Design review of the part built by this model. Coordinates are the model's own, in mm. Face numbers are marked on the shaded views. A direction names the side the tool comes from. Give positions to 0.01 mm unless a question says otherwise; leave off trailing zeros. Order: outer loops, then holes, each group sorted by start corner. A loop starts at its lowest first (then second) coordinate and runs counter-clockwise, first axis right, second up. Notation, with made-up numbers: (2.25, 65) -> (36.25, 65) arc R18 cw to (36.25, 91) -> close; hole circle Ø4 at (66.25, -12). An arc over 180 degrees is marked (long way). Answer in a Markdown table with one row per item. Add a question column.
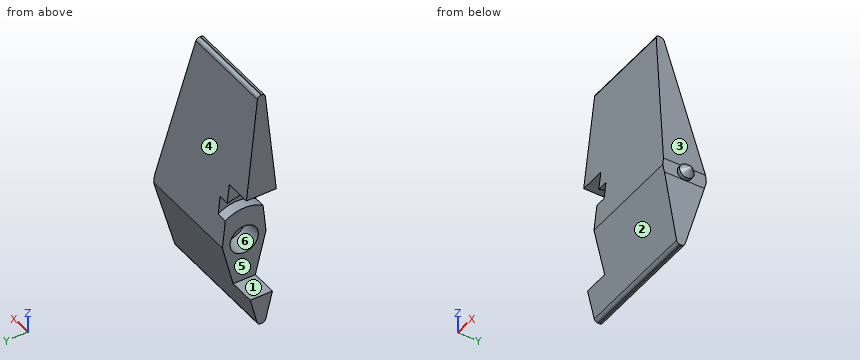
```python
from build123d import *

# Parameters (mm, degrees)
SKETCH_1_3_R                  = 1.95
CUT_EXTRUDE_1_DEPTH           = 6.5
CUT_EXTRUDE_2_DEPTH           = 30.951001802
CUT_EXTRUDE_2_DEPTH_BACK      = 30.951001802
SKETCH_4_W                    = 3.6
SKETCH_4_H                    = 14.9
SKETCH_5_W                    = 1.5
SKETCH_5_H                    = 2.1
CUT_REVOLVE_1_ANGLE           = 40
CUT_REVOLVE_1_OTHER_WAY_ANGLE = 40
SKETCH_3_3_R                  = 1
EXTRUDE_1_DEPTH               = 1.5
CHAMFER_1_SIZE                = 1
CUT_EXTRUDE_3_DEPTH           = 31.875759187
CUT_EXTRUDE_3_DEPTH_BACK      = 31.875759187
FILLET_1_R                    = 0.5


with BuildPart() as part:
    # Эскиз1 → По сечениям1 section 0
    with BuildSketch(Plane(origin=(0, 0, 0), x_dir=(0, 0, -1), z_dir=(1, 0, 0))):
        with BuildLine():
            Line((-23.75, -0.5), (-23.75, 0.5))
            Line((-23.75, 0.5), (0, 3))
            Line((0, 3), (10, 0.5))
            Line((10, 0.5), (10, -0.5))
            Line((10, -0.5), (0, -3))
            Line((0, -3), (-23.75, -0.5))
        make_face()
    # Эскиз3 → По сечениям1 section 1
    with BuildSketch(Plane(origin=(18, 0, 0), x_dir=(0, 0, -1), z_dir=(1, 0, 0))):
        with BuildLine():
            Line((0, 3), (10, 0.5))
            Line((10, 0.5), (10, -0.5))
            Line((10, -0.5), (0, -3))
            Line((0, -3), (-23.75, -0.5))
            Line((-23.75, -0.5), (-23.75, 0.5))
            Line((-23.75, 0.5), (0, 3))
        make_face()
    loft()

    # Эскиз1<3> → Вырез-Вытянуть1 (cut)
    with BuildSketch(Plane(origin=(0, 0, 0), x_dir=(0, 0, -1), z_dir=(1, 0, 0))):
        with Locations(Location((0, 0, 0), (0, 0, 180))):
            Circle(SKETCH_1_3_R)
    extrude(amount=CUT_EXTRUDE_1_DEPTH, mode=Mode.SUBTRACT)

    # Эскиз4 → Вырез-Вытянуть2 (cut, two sides: drawn at the far end of the back side and taken through both)
    with BuildSketch(Plane(origin=(0, 0, 0), x_dir=(1, 0, 0), z_dir=(0, 1, 0)).offset(-CUT_EXTRUDE_2_DEPTH_BACK)):
        with Locations((1.8, -1.55)):
            Rectangle(SKETCH_4_W, SKETCH_4_H)
    extrude(amount=CUT_EXTRUDE_2_DEPTH + CUT_EXTRUDE_2_DEPTH_BACK, mode=Mode.SUBTRACT)

    # Эскиз5 → Вырез-Повернуть1 (revolve, cut)
    with BuildSketch(Plane(origin=(0, 0, 0), x_dir=(1, 0, 0), z_dir=(0, 1, 0))):
        with Locations((4.35, -5.7)):
            Rectangle(SKETCH_5_W, SKETCH_5_H)
    revolve(axis=Axis((6.5, 0, 0), (-1, 0, 0)), revolution_arc=CUT_REVOLVE_1_ANGLE, mode=Mode.SUBTRACT)

    # Эскиз5 → Вырез-Повернуть1 other way (revolve, cut)
    with BuildSketch(Plane(origin=(0, 0, 0), x_dir=(1, 0, 0), z_dir=(0, 1, 0))):
        with Locations((4.35, -5.7)):
            Rectangle(SKETCH_5_W, SKETCH_5_H)
    revolve(axis=Axis((6.5, 0, 0), (1, 0, 0)), revolution_arc=CUT_REVOLVE_1_OTHER_WAY_ANGLE, mode=Mode.SUBTRACT)

    # Эскиз3<3> → Бобышка-Вытянуть1 (add)
    with BuildSketch(Plane(origin=(18, 0, 0), x_dir=(0, 0, -1), z_dir=(1, 0, 0))):
        with Locations(Location((0, 0, 0), (0, 0, 180))):
            Circle(SKETCH_3_3_R)
    extrude(amount=EXTRUDE_1_DEPTH)

    # Фаска1
    chamfer_1_edges = [part.edges().sort_by_distance(p)[0] for p in [
        (19.5, 0, -1),
    ]]
    chamfer(chamfer_1_edges, length=CHAMFER_1_SIZE)

    # Эскиз6 → Вырез-Вытянуть3 (cut, two sides: drawn at the far end of the back side and taken through both)
    with BuildSketch(Plane(origin=(0, 0, 0), x_dir=(1, 0, 0), z_dir=(0, 1, 0)).offset(-CUT_EXTRUDE_3_DEPTH_BACK)):
        Polygon((18, 10), (17.2, 10), (18, 1), align=None)
        Polygon((12.8, -23.75), (18, -23.75), (18, -1), align=None)
    extrude(amount=CUT_EXTRUDE_3_DEPTH + CUT_EXTRUDE_3_DEPTH_BACK, mode=Mode.SUBTRACT)

    # Скругление1
    fillet_1_edges = [part.edges().sort_by_distance(p)[0] for p in [
        (6.4, 0.5, 23.75),
        (6.4, -0.5, 23.75),
        (8.6, 0.5, -10),
        (8.6, -0.5, -10),
    ]]
    fillet(fillet_1_edges, radius=FILLET_1_R)


solid = part.part
```
1) Add section A-A, the plane z = 3.5. Write out the cut boundary in (x, y), and give its area (3 significant figures).
2) Machinability: for the marked faces 4, 5 and 6, which of the approach directions +Z, -Z, +X, -X, +Y, -Y give a long, thin tool a straight path to every point of the face, cutting with its end or side? Answer none if there is none.
3) Add section B-B, the plane z = 21.5. Write out the cut boundary in (x, y).
4) For L1, parallel to Y at x = 5.2, z = 0; L2, parallel to Z at x = 1.75, y = 0; L3, parallel to Y at x = 13.75, z = 19, list the stretches that pass through material, from the lowest coordinate up.
5) Clearance check with flat-ended pins moving along their axes: P1, Ø3, axis at x = 13, z = 2, coming from the +Y side; P2, Ø3, axis at y = 1, z = 0.5, coming from the -X side; P3, Ø1.6, axis at y = -2, z = 0, coming from the +X side. State where each tip first meets the part, or that it passes through.
6) Mouldability with a two-part tool opening along Z and no side actions: class the marked faces 1, 2 and 3 as +Z half, -Z half, draft (parallel to the pull), parting line (faces both ways), or undercut.
Verdict:
| question | item | result |
|---|---|---|
| 1 | outline | (3.6, -2.63) -> (17.43, -2.63) -> (17.43, 2.63) -> (3.6, 2.63) -> close |
| 1 | area | 72.8 mm2 |
| 2 | face 4 | +Z, +X, -X, +Y |
| 2 | face 5 | -X, +Y, -Y |
| 2 | face 6 | -X |
| 3 | outline | (0, -0.74) -> (13.31, -0.74) -> (13.31, 0.74) -> (0, 0.74) -> close |
| 4 | L1 | y = -3 to -1.95, 1.95 to 3 |
| 4 | L2 | z = -10 to -5.9, 9 to 23.75 |
| 4 | L3 | y = -1 to 1 |
| 5 | P1 | stops at y = 2.95 |
| 5 | P2 | stops at x = 3.6 |
| 5 | P3 | stops at x = 18 |
| 6 | face 1 | undercut |
| 6 | face 2 | -Z half |
| 6 | face 3 | +Z half |
